```python
from build123d import *

# Parameters (mm, degrees)
SKETCH2_OUTSIDE_W               = 13.34
SKETCH2_OUTSIDE_H               = 13.34
CUT_EXTRUDE1_DEPTH              = 17.856007831
M4X0_7_TAPPED_HOLE1_D           = 3.3
M4X0_7_TAPPED_HOLE1_DEPTH       = 14.5
M4X0_7_TAPPED_HOLE1_CBORE_D     = 4
M4X0_7_TAPPED_HOLE1_CBORE_DEPTH = 13.1
M4X0_7_TAPPED_HOLE1_TIP         = 0.991420021
M4X0_7_TAPPED_HOLE2_D           = 3.3
M4X0_7_TAPPED_HOLE2_DEPTH       = 12.5
M4X0_7_TAPPED_HOLE2_CBORE_D     = 4
M4X0_7_TAPPED_HOLE2_CBORE_DEPTH = 11.1
M4X0_7_TAPPED_HOLE2_TIP         = 0.991420021


with BuildPart() as part:
    # Sketch1 → Revolve1 (revolve)
    with BuildSketch(Plane(origin=(0, 0, 0), x_dir=(0, 0, -1), z_dir=(1, 0, 0)), mode=Mode.PRIVATE) as revolve1_sk:
        Polygon((-8, 0), (-8, 3), (-7.566987298, 3.75), (7.566987298, 3.75), (8, 3), (8, 0), align=None)
    revolve(revolve1_sk.sketch.rotate(Axis((0, 0, 5.584882278), (0, 0, -1)), 180), axis=Axis((0, 0, 5.584882278), (0, 0, -1)))

    # Sketch2 outside → Cut-Extrude1 (cut, through all)
    with BuildSketch(Plane.XY.offset(8)):
        Rectangle(SKETCH2_OUTSIDE_W, SKETCH2_OUTSIDE_H)
        Polygon((1.732050808, -3), (3.464101615, 0), (1.732050808, 3), (-1.732050808, 3), (-3.464101615, 0), (-1.732050808, -3), align=None, mode=Mode.SUBTRACT)
    extrude(amount=-CUT_EXTRUDE1_DEPTH, mode=Mode.SUBTRACT)

    # M4x0.7 Tapped Hole1
    with Locations(Plane.XY.offset(8)):
        with Locations((0, 0)):
            CounterBoreHole(M4X0_7_TAPPED_HOLE1_D / 2, M4X0_7_TAPPED_HOLE1_CBORE_D / 2, M4X0_7_TAPPED_HOLE1_CBORE_DEPTH, depth=M4X0_7_TAPPED_HOLE1_DEPTH)
            with Locations((0, 0, -(M4X0_7_TAPPED_HOLE1_DEPTH + M4X0_7_TAPPED_HOLE1_TIP / 2))):  # 118° drill point
                Cone(0, M4X0_7_TAPPED_HOLE1_D / 2, M4X0_7_TAPPED_HOLE1_TIP, mode=Mode.SUBTRACT)

    # M4x0.7 Tapped Hole2
    with Locations(Plane(origin=(0, 0, -8), x_dir=(-1, 0, 0), z_dir=(0, 0, -1))):
        with Locations((0, 0)):
            CounterBoreHole(M4X0_7_TAPPED_HOLE2_D / 2, M4X0_7_TAPPED_HOLE2_CBORE_D / 2, M4X0_7_TAPPED_HOLE2_CBORE_DEPTH, depth=M4X0_7_TAPPED_HOLE2_DEPTH)
            with Locations((0, 0, -(M4X0_7_TAPPED_HOLE2_DEPTH + M4X0_7_TAPPED_HOLE2_TIP / 2))):  # 118° drill point
                Cone(0, M4X0_7_TAPPED_HOLE2_D / 2, M4X0_7_TAPPED_HOLE2_TIP, mode=Mode.SUBTRACT)


solid = part.part
```
Design review of the part built by this model. Coordinates are the model's own, in mm. Coordinates: 2 decimals unless noted, no trailing zeros. Order: outer loops, then holes, each group sorted by start corner. A loop starts at its lowest first (then second) coordinate and runs counter-clockwise, first axis right, second up. Notation, with made-up numbers: M 53.5,77.5 L 74.5,77.5 A18 cw 74.5,82.5 Z; hole C 0,-3.75 d1. An arc over 180 degrees is marked long. Answer as a JSON object with one key per item and string values. Group by question number.
1) Add section A-A, the plane z = -0.25. Write out the cut boundary in (x, y).
2) Wall thickness on L1, parallel to Y at x = -1, z = -3.5; L2, parallel to Y at x = 0, z = 1.75; L3, parallel to X at y = 1.5, z = -4.25: over which ranges is each line inside the solid? List them lowest first.
3) Mouldability with a two-part tool opening along X and no side actions: class faces 1 (the flat face through (2.6, 1.5, 0.1)), 2 (the flat face through (-2.6, 1.5, 0.1)), 3 (the cylindrical face through (0, 2, 0)) as pulls with the +X half, pulls with the -X half, needs draft (parallel to the pull), parting line crosses it, or undercut.
Computed values:
{
 "1": {"outline": "M -3.46,0 L -1.73,-3 L 1.73,-3 L 3.46,0 L 1.73,3 L -1.73,3 Z; hole C 0,0 d4"},
 "2": {"L1": "y = -3 to -1.73, 1.73 to 3", "L2": "y = -3 to -2, 2 to 3", "L3": "x = -2.6 to -1.32, 1.32 to 2.6"},
 "3": {"face 1": "pulls with the +X half", "face 2": "pulls with the -X half", "face 3": "undercut"}
}
